Could you check a few things on this drawing? It's one solid part, dimensions in mm from its lowest x, y, z. Give positions to 0.01 mm unless a question says otherwise; leave off trailing zeros. Write each loop counter-clockwise with the first axis right and the second up, starting at its lowest first coordinate (ties: lowest second). Pieces come first, ordered by that corner, then holes. Notation, with made-up numbers: M -15.75,-5 L 28.25,-5 A28 cw 28.25,14 Z; hole C 18.5,13 d8. An arc over 180 degrees is marked long. Write each question's results on one line, items separated by ' | '. Start each with the question number.
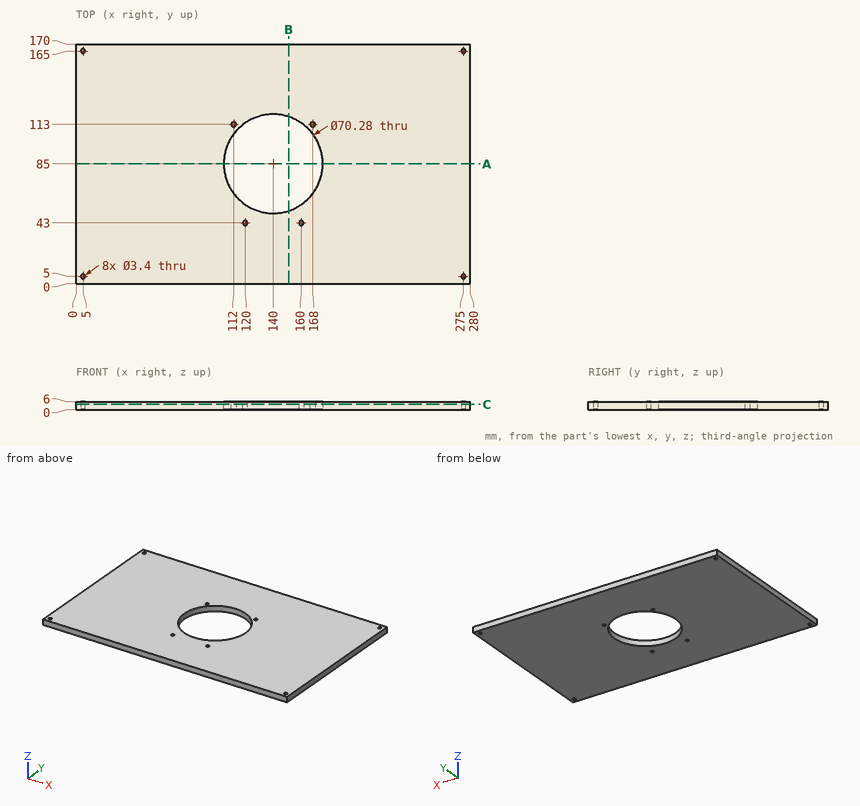
Q1. I'm going to push a flat-ended pin straight in: P1, Ø2, axis at x = 134.5, z = 5.5, coming from the -Y side. Where does the tip first touch, or does it pass through?
Q2. If we section it at B-B (x = 151): Please give me the cut outline in (y, z), plus the area to 3 significant figures.
Q3. If we section it at A-A (y = 85): Please give me the cut outline in (x, z).
Q4. Please list where these lines run through material, in increasing order: line 1 (X direction, y = 5, z = 3.8); line 2 (Y direction, x = 275, z = 2.5); line 3 (X direction, y = 43, z = 3.4). Write a range as [from, to].
Q5. If we section it at C-C (z = 3.95): Count the separate pieces of the cut face and the enclosed holes in it, plus the area to 3 significant figures.
Determined:
1) P1: stops at y = 0
2) outline: M 0,0 L 51.63,0 L 51.63,6 L 0,6 Z; M 118.37,0 L 170,0 L 170,6 L 118.37,6 Z | area: 620 mm²
3) outline: M 0,0 L 104.86,0 L 104.86,6 L 0,6 Z; M 175.14,0 L 280,0 L 280,6 L 175.14,6 Z
4) line 1: x = [0, 3.3], [6.7, 273.3], [276.7, 280] | line 2: y = [0, 3.3], [6.7, 163.3], [166.7, 170] | line 3: x = [0, 118.3], [121.7, 158.3], [161.7, 280]
5) separate pieces: 1 | enclosed holes: 9 | area: 43,600 mm²
